from build123d import *
from OCP.BRepFilletAPI import BRepFilletAPI_MakeChamfer

# Parameters (mm, degrees)
SKETCH_1_R          = 55
EXTRUDE_1_DEPTH     = 5
SKETCH_2_R          = 49.9
EXTRUDE_2_DEPTH     = 5
SKETCH7_W           = 51.010205144
SKETCH7_H           = 50
BOSS_EXTRUDE2_DEPTH = 5
SKETCH_3_W          = 35
SKETCH_3_H          = 30
EXTRUDE_3_DEPTH     = 25
SKETCH_4_W          = 20.2
SKETCH_4_H          = 10.3
CUT_EXTRUDE_1_DEPTH = 125.599357944
SKETCH_5_R          = 4.1
CUT_EXTRUDE_2_DEPTH = 117.833214455
CHAMFER1_SIZE       = 2
CHAMFER1_SIZE2      = 0.535898385
SKETCH2_W           = 35
SKETCH2_H           = 30
CUT_EXTRUDE1_DEPTH  = 12.5
BOSS_EXTRUDE1_START = -2
SKETCH4_W           = 70
SKETCH4_H           = 20
BOSS_EXTRUDE1_DEPTH = 5.35
SKETCH5_R           = 4.15
CUT_EXTRUDE2_DEPTH  = 116.154776293
SKETCH9_R           = 4.15
BOSS_EXTRUDE3_DEPTH = 5
CHAMFER3_SIZE       = 2
CHAMFER3_SIZE2      = 0.535898385
CUT_EXTRUDE3_DEPTH  = 6.5
CHAMFER2_SIZE       = 1
CHAMFER2_SIZE2      = 2.747477419
CHAMFER4_SIZE       = 10.579618843
CHAMFER4_SIZE_2     = 60


with BuildPart() as part:
    # Эскиз1 → Бобышка-Вытянуть1 (new body)
    with BuildSketch(Plane(origin=(0, 0, 0), x_dir=(1, 0, 0), z_dir=(0, 1, 0))):
        with Locations(Location((0, 0, 0), (0, 0, 270))):
            Circle(SKETCH_1_R)
    extrude(amount=EXTRUDE_1_DEPTH)

    # Эскиз2 → Бобышка-Вытянуть2 (add)
    with BuildSketch(Plane(origin=(0, 5, 0), x_dir=(1, 0, 0), z_dir=(0, 1, 0))):
        with Locations(Location((0, 0, 0), (0, 0, 270))):
            Circle(SKETCH_2_R)
    extrude(amount=EXTRUDE_2_DEPTH)

    # Sketch7 → Boss-Extrude2 (add)
    with BuildSketch(Plane.XZ):
        with Locations((74.494897428, 0)):
            Rectangle(SKETCH7_W, SKETCH7_H)
    extrude(amount=-BOSS_EXTRUDE2_DEPTH)

    # Эскиз3 → Бобышка-Вытянуть3 (add)
    with BuildSketch(Plane.XZ):
        with Locations((62.5, 0)):
            Rectangle(SKETCH_3_W, SKETCH_3_H)
    extrude(amount=EXTRUDE_3_DEPTH)

    # Эскиз4 → Вырез-Вытянуть1 (cut, through all)
    with BuildSketch(Plane.XY.offset(15)):
        with Locations((62.5, -12.5)):
            Rectangle(SKETCH_4_W, SKETCH_4_H)
    extrude(amount=-CUT_EXTRUDE_1_DEPTH, mode=Mode.SUBTRACT)

    # Эскиз5 → Вырез-Вытянуть2 (cut, through all)
    with BuildSketch(Plane.XZ):
        with Locations(Location((33.234018716, -33.234018716, 0), (0, 0, 270))):
            Circle(SKETCH_5_R)
        with Locations(Location((-33.234018716, -33.234018716, 0), (0, 0, 270))):
            Circle(SKETCH_5_R)
        with Locations(Location((-33.234018716, 33.234018716, 0), (0, 0, 270))):
            Circle(SKETCH_5_R)
        with Locations(Location((33.234018716, 33.234018716, 0), (0, 0, 270))):
            Circle(SKETCH_5_R)
    extrude(amount=-CUT_EXTRUDE_2_DEPTH, mode=Mode.SUBTRACT)

    # Chamfer1: one chamfer whose edges measure the first distance from different faces: ONE call of the kernel's chamfer builder (chamfer() names one face for all edges)
    chamfer1_edges_1 = [part.edges().sort_by_distance(p)[0] for p in [
        (0, 10, -49.9),
    ]]
    chamfer1_side_1 = [part.faces().sort_by_distance(p)[0] for p in [
        (0, 7.5, -49.9),
    ]]
    chamfer1_edges_2 = [part.edges().sort_by_distance(p)[0] for p in [
        (-49.9, 10, 0),
    ]]
    chamfer1_side_2 = [part.faces().sort_by_distance(p)[0] for p in [
        (-49.9, 7.5, 0),
    ]]
    chamfer1_edges_3 = [part.edges().sort_by_distance(p)[0] for p in [
        (0, 10, 49.9),
    ]]
    chamfer1_side_3 = [part.faces().sort_by_distance(p)[0] for p in [
        (0, 7.5, 49.9),
    ]]
    chamfer1_edges_4 = [part.edges().sort_by_distance(p)[0] for p in [
        (49.9, 10, 0),
    ]]
    chamfer1_side_4 = [part.faces().sort_by_distance(p)[0] for p in [
        (49.9, 7.5, 0),
    ]]
    chamfer1 = BRepFilletAPI_MakeChamfer(part.part.solid().wrapped)
    for e in chamfer1_edges_1:
        chamfer1.Add(CHAMFER1_SIZE, CHAMFER1_SIZE2, e.wrapped, chamfer1_side_1[0].wrapped)  # the first distance lies on this face
    for e in chamfer1_edges_2:
        chamfer1.Add(CHAMFER1_SIZE, CHAMFER1_SIZE2, e.wrapped, chamfer1_side_2[0].wrapped)  # the first distance lies on this face
    for e in chamfer1_edges_3:
        chamfer1.Add(CHAMFER1_SIZE, CHAMFER1_SIZE2, e.wrapped, chamfer1_side_3[0].wrapped)  # the first distance lies on this face
    for e in chamfer1_edges_4:
        chamfer1.Add(CHAMFER1_SIZE, CHAMFER1_SIZE2, e.wrapped, chamfer1_side_4[0].wrapped)  # the first distance lies on this face
    add(Compound.cast(chamfer1.Shape()), mode=Mode.REPLACE)

    # Sketch2 → Cut-Extrude1 (cut)
    with BuildSketch(Plane.XZ.offset(25)):
        with Locations((62.5, 0)):
            Rectangle(SKETCH2_W, SKETCH2_H)
    extrude(amount=-CUT_EXTRUDE1_DEPTH, mode=Mode.SUBTRACT)

    # Sketch4 → Boss-Extrude1 (add)
    with BuildSketch(Plane.XZ.offset(7.35).offset(BOSS_EXTRUDE1_START)):
        with Locations((62.5, 0)):
            Rectangle(SKETCH4_W, SKETCH4_H)
    extrude(amount=-BOSS_EXTRUDE1_DEPTH)

    # Sketch5 → Cut-Extrude2 (cut, through all)
    with BuildSketch(Plane.XZ.offset(5.35)):
        with Locations((87.5, 0)):
            Circle(SKETCH5_R)
        with Locations((37.5, 0)):
            Circle(SKETCH5_R)
    extrude(amount=-CUT_EXTRUDE2_DEPTH, mode=Mode.SUBTRACT)

    # Sketch9 → Boss-Extrude3 (add)
    # profile 1 of 2: a face of its own
    with BuildSketch(Plane(origin=(0, 5, 0), x_dir=(1, 0, 0), z_dir=(0, 1, 0))):
        with Locations((37.5, 0)):
            Circle(SKETCH9_R)
    # profile 2 of 2: a face of its own
    with BuildSketch(Plane(origin=(0, 5, 0), x_dir=(1, 0, 0), z_dir=(0, 1, 0))):
        with BuildLine():
            Line((49.389794856, -25), (100, -25))
            Line((100, -25), (100, 25))
            Line((100, 25), (49.389794856, 25))
            ThreePointArc((49.389794856, 25), (55.356588008, 0), (49.389794856, -25))
        make_face()
        with Locations((87.5, 0)):
            Circle(SKETCH9_R, mode=Mode.SUBTRACT)
    extrude(amount=BOSS_EXTRUDE3_DEPTH)

    # Chamfer3
    chamfer3_edges = [part.edges().sort_by_distance(p)[0] for p in [
        (55.356588008, 10, 0),
    ]]
    chamfer3_side = [part.faces().sort_by_distance(p)[0] for p in [
        (55.356588008, 7.5, 0),
    ]]
    chamfer(chamfer3_edges, length=CHAMFER3_SIZE, length2=CHAMFER3_SIZE2, reference=chamfer3_side[0])

    # Sketch6 → Cut-Extrude3 (cut)
    with BuildSketch(Plane(origin=(0, 10, 0), x_dir=(1, 0, 0), z_dir=(0, 1, 0))):
        Polygon((43.995190528, 3.75), (37.5, 7.5), (31.004809472, 3.75), (31.004809472, -3.75), (37.5, -7.5), (43.995190528, -3.75), align=None)
        Polygon((93.995190528, 3.75), (87.5, 7.5), (81.004809472, 3.75), (81.004809472, -3.75), (87.5, -7.5), (93.995190528, -3.75), align=None)
    extrude(amount=-CUT_EXTRUDE3_DEPTH, mode=Mode.SUBTRACT)

    # Chamfer2: one chamfer whose edges measure the first distance from different faces: ONE call of the kernel's chamfer builder (chamfer() names one face for all edges)
    chamfer2_edges_1 = [part.edges().sort_by_distance(p)[0] for p in [
        (43.995190528, 10, 0),
        (40.747595264, 10, -5.625),
        (34.252404736, 10, -5.625),
        (31.004809472, 10, 0),
        (34.252404736, 10, 5.625),
        (40.747595264, 10, 5.625),
    ]]
    chamfer2_side_1 = [part.faces().sort_by_distance(p)[0] for p in [
        (-0.7474754, 10, 0),
    ]]
    chamfer2_edges_2 = [part.edges().sort_by_distance(p)[0] for p in [
        (93.995190528, 10, 0),
        (90.747595264, 10, -5.625),
        (84.252404736, 10, -5.625),
        (81.004809472, 10, 0),
        (84.252404736, 10, 5.625),
        (90.747595264, 10, 5.625),
    ]]
    chamfer2_side_2 = [part.faces().sort_by_distance(p)[0] for p in [
        (76.23589774, 10, 0),
    ]]
    chamfer2 = BRepFilletAPI_MakeChamfer(part.part.solid().wrapped)
    for e in chamfer2_edges_1:
        chamfer2.Add(CHAMFER2_SIZE, CHAMFER2_SIZE2, e.wrapped, chamfer2_side_1[0].wrapped)  # the first distance lies on this face
    for e in chamfer2_edges_2:
        chamfer2.Add(CHAMFER2_SIZE, CHAMFER2_SIZE2, e.wrapped, chamfer2_side_2[0].wrapped)  # the first distance lies on this face
    add(Compound.cast(chamfer2.Shape()), mode=Mode.REPLACE)

    # Chamfer4
    # the kernel refuses this chamfer: 60, 10.579618843 mm, written as the material it takes off along each edge
    with BuildSketch(Plane(origin=(100, 165.912327785, -25), x_dir=(0.21013876076743138, 0, 0.9776715712462587), z_dir=(0, -1, 0))) as chamfer4_piece_1_section:
        Polygon((CHAMFER4_SIZE * 0.977671571201, CHAMFER4_SIZE * 0.210138760758), (-CHAMFER4_SIZE_2 * 0.210138760767, CHAMFER4_SIZE_2 * 0.977671571246), (0, 0), align=None)
    chamfer4_piece_1 = extrude(amount=321.824655571, mode=Mode.PRIVATE)
    chamfer4_piece_1 = chamfer4_piece_1 - Plane(origin=(0, 7.498692245, 0), x_dir=(0, 0, 1), z_dir=(0, -1, 0)) * Cylinder(55, 879, mode=Mode.PRIVATE)
    add(chamfer4_piece_1, mode=Mode.SUBTRACT)
    with BuildSketch(Plane(origin=(100, -155.912327785, 25), x_dir=(-0.9999776716360547, 0, 0.006682531656101301), z_dir=(0, 1, 0))) as chamfer4_piece_2_section:
        Polygon((CHAMFER4_SIZE_2 * 0.999977671636, -CHAMFER4_SIZE_2 * 0.0066825316561), (-CHAMFER4_SIZE * 0.00668253165579, -CHAMFER4_SIZE * 0.99997767159), (0, 0), align=None)
    chamfer4_piece_2 = extrude(amount=321.824655571, mode=Mode.PRIVATE)
    chamfer4_piece_2 = chamfer4_piece_2 - Plane(origin=(0, 2.5, 0), x_dir=(0, 0, 1), z_dir=(0, -1, 0)) * Cylinder(55, 884, mode=Mode.PRIVATE)
    add(chamfer4_piece_2, mode=Mode.SUBTRACT)


solid = part.part
Here's how the part is built. I have some questions about the finished solid (model axes, mm). A direction names the side the tool comes from. Coordinates: 2 decimals unless noted, no trailing zeros. Write each loop counter-clockwise with the first axis right and the second up, starting at its lowest first coordinate (ties: lowest second). Pieces come first, ordered by that corner, then holes.
1) If we section it at C-C (z = 0): Count the separate pieces of the cut face and the enclosed holes in it, plus the area to 3 significant figures.
Filled in:
separate pieces: 3
enclosed holes: 0
area: 1,700 mm2
2) Thinking about a two-plate mould opening in Z: for faces 5 (the face through (75, 10, 0)), 6 (the face through (0.502, 9.681, -49.447)), 7 (the face through (81.005, 5, 0)), which applies, +Z half, -Z half, draft (parallel to the pull), parting line (faces both ways), or undercut?
Filled in:
face 5: draft
face 6: -Z half
face 7: undercut
3) If we section it at B-B (x = 0): List the corners of the cut face in (y, z) for me.
Filled in:
outline: (0, -55) - (5, -55) - (5, -49.9) - (8, -49.9) - (10, -49.36) - (10, 49.36) - (8, 49.9) - (5, 49.9) - (5, 55) - (0, 55) - close
4) If we section it at A-A (y = -9.75): List the corners of the cut face in (x, z) for me, plus the area to 3 significant figures.
Filled in:
outline: (45, -15) - (52.4, -15) - (52.4, 15) - (45, 15) - close; (72.6, -15) - (80, -15) - (80, 15) - (72.6, 15) - close
area: 444 mm2
5) I'm going to push flat-ended pins straight in: pin 1 (12 mm diameter, centred on x = 18.5, z = -23, fed in from -Y); pin 2 (11 mm diameter, centred on x = 87.5, z = 0, fed in from +Y); pin 3 (6 mm diameter, centred on x = 69.5, y = 5.5, fed in from +Z). Where does each tip first touch, or does it pass through?
Filled in:
pin 1: stops at y = 0
pin 2: stops at y = 3.5
pin 3: stops at z = 20.33
6) Which directions (+Z, -Z, +X, -X, +Y, -Y) give clear straight access to the entire face, cutting with the end or side of a thin tool? Please do faces 1 (the face through (89, -3, 10)), 2 (the face through (36, -3, -10)), 3 (the face through (83.95, 8.61, 6.02)), 4 (the face through (0.507, 6.479, -49.897)).
Filled in:
face 1: +Z, +X, -Y
face 2: -Z, -X, -Y
face 3: +Y
face 4: -Z, +Y
7) If I drill on line 1 (Z direction, x = 37.5, y = -0.25); line 2 (X direction, y = 5.25, z = 5.5); line 3 (X direction, y = 2.5, z = -33), over which ranges is the centre line in solid material (lowest first)?
Filled in:
line 1: z = -10 to -4.15, 4.15 to 10
line 2: x = -49.6 to 34.04, 40.96 to 49.6, 55.08 to 84.04, 90.96 to 100
line 3: x = -44 to -37.33, -29.14 to 29.14, 37.33 to 44
